Work out the finished part from the listing and answer in its coordinate system (mm). A direction names the side the tool comes from. Round coordinates to 2 decimals unless told otherwise and drop trailing zeros. Order: outer loops, then holes, each group sorted by start corner. A loop starts at its lowest first (then second) coordinate and runs counter-clockwise, first axis right, second up. Notation, with made-up numbers: (35, 46) -> (85, 46) arc R28 cw to (85, 73) -> close; hole circle Ø9 at (4.5, 68). An arc over 180 degrees is marked (long way). Use a Markdown table: item, result. Add a question column.
Item 1: Find the intervals of material crossed by L1, parallel to Z at x = -39, y = -22; L2, parallel to Z at x = -20, y = -17.78; L3, parallel to Z at x = -8.5, y = -53, in increasing order. Write a range as [from, to].
Item 2: A cutting plane is placed at B-B, the plane z = -53.34. Give the number of separate pieces and of enclosed holes in the cut face, plus the area to 3 significant figures.
Item 3: For a pull along X with two mould halves and no side action, classify faces 1 (the flat face through (-38, -28.702, 75)), 2 (the flat face through (-4, -60.757, 1)), 3 (the flat face through (-15.748, -48, -51)), 4 (the cylindrical face through (-41.253, -14.406, 75.323)) as +X half, -X half, draft (parallel to the pull), parting line (faces both ways), or undercut.
Item 4: A cutting plane is placed at A-A, the plane x = -13. Determine the outline of the cut face in (y, z), plus the area to 3 significant figures.
Item 5: A tool of negligible diameter and unlimited length cuts with its end or side. For faces 5 (the cylindrical face through (-8.09, -16.23, -57.08)), 6 (the cylindrical face through (-41.25, -14.41, -69.1)), 7 (the flat face through (-1.524, -30, 78)), from which of +Z, -Z, +X, -X, +Y, -Y can it reach the whole face along a straight path? Write none if from no direction.
Item 6: A cutting plane is placed at C-C, the plane y = -32. Determine the outline of the cut face in (x, z) (3 decimals).
Item 7: Flat-ended cylindrical pins translate along their axes: P1, Ø17, axis at y = -27, z = 72.5, coming from the +X side; P2, Ø9, axis at x = -39.497, z = -74.676, coming from the -Y side; P3, Ø6.5, axis at y = -17.78, z = 48.26, coming from the +X side; P4, Ø1, axis at x = -45, z = 49, coming from the -Y side. Find the tip coordinate at first contact, or state that the pin passes through.
Item 8: A cutting plane is placed at D-D, the plane z = -21.5. Determine the outline of the cut face in (x, y).
from build123d import *

# Parameters (mm, degrees)
EXTRUDE1_DEPTH                              = 95.25
TAPPED_HOLE_FOR_3_8_16_HELICOIL1_AT_2_COUNT = 2
TAPPED_HOLE_FOR_3_8_16_HELICOIL1_AT_2_PITCH = 38.1
TAPPED_HOLE_FOR_3_8_16_HELICOIL1_AT_3_COUNT = 2
TAPPED_HOLE_FOR_3_8_16_HELICOIL1_AT_3_PITCH = 106.3244
TAPPED_HOLE_FOR_3_8_16_HELICOIL1_AT_4_COUNT = 2
TAPPED_HOLE_FOR_3_8_16_HELICOIL1_AT_4_PITCH = 144.4244
TAPPED_HOLE_FOR_1_4_20_HELICOIL1_AT_2_COUNT = 2
TAPPED_HOLE_FOR_1_4_20_HELICOIL1_AT_2_PITCH = 33.02
TAPPED_HOLE_FOR_1_4_20_HELICOIL1_AT_3_COUNT = 2
TAPPED_HOLE_FOR_1_4_20_HELICOIL1_AT_3_PITCH = 106.831083492
TAPPED_HOLE_FOR_1_4_20_HELICOIL1_AT_4_COUNT = 2
TAPPED_HOLE_FOR_1_4_20_HELICOIL1_AT_4_PITCH = 101.6
F_1_4_0_25_DIAMETER_HOLE1_D                 = 6.35
F_1_4_0_25_DIAMETER_HOLE1_CSINK_D           = 7.62
F_1_4_0_25_DIAMETER_HOLE1_CSINK_ANGLE       = 90
SKETCH20_W                                  = 76.2
SKETCH20_H                                  = 60.757213881
SKETCH20_W_2                                = 29.21
SKETCH20_W_3                                = 34.29
EXTRUDE2_DEPTH                              = 1.524


with BuildPart() as part:
    # Sketch13 → Extrude1 (new body, symmetric)
    with BuildSketch(Plane.XY):
        Polygon((0, -60.757213881), (-6.35, -60.757213881), (-76.2, -35.333893017), (-76.2, 0), (0, 0), align=None)
    extrude(amount=EXTRUDE1_DEPTH, both=True)

    # Sketch14 → Tapped Hole for 3/8-16 Helicoil1 (revolve, cut)
    with BuildSketch(Plane(origin=(-39.497, 0, 69.7484), x_dir=(0, 0, 1), z_dir=(1, 0, 0))):
        Polygon((0, 0), (0, 60.757213881), (5.0419, 60.757213881), (5.0419, 28.702), (5.84454, 28.702), (5.84454, 0.50546), (6.35, 0), align=None)
    tapped_hole_for_3_8_16_helicoil1 = revolve(axis=Axis((-39.497, 6.35, 69.7484), (0, -1, 0)), mode=Mode.SUBTRACT)

    # Tapped Hole for 3/8-16 Helicoil1 at 2: Tapped Hole for 3/8-16 Helicoil1 ×2
    with Locations(*[(0, 0, -i * TAPPED_HOLE_FOR_3_8_16_HELICOIL1_AT_2_PITCH) for i in range(1, TAPPED_HOLE_FOR_3_8_16_HELICOIL1_AT_2_COUNT)]):
        add(tapped_hole_for_3_8_16_helicoil1, mode=Mode.SUBTRACT)

    # Tapped Hole for 3/8-16 Helicoil1 at 3: Tapped Hole for 3/8-16 Helicoil1 ×2
    with Locations(*[(0, 0, -i * TAPPED_HOLE_FOR_3_8_16_HELICOIL1_AT_3_PITCH) for i in range(1, TAPPED_HOLE_FOR_3_8_16_HELICOIL1_AT_3_COUNT)]):
        add(tapped_hole_for_3_8_16_helicoil1, mode=Mode.SUBTRACT)

    # Tapped Hole for 3/8-16 Helicoil1 at 4: Tapped Hole for 3/8-16 Helicoil1 ×2
    with Locations(*[(0, 0, -i * TAPPED_HOLE_FOR_3_8_16_HELICOIL1_AT_4_PITCH) for i in range(1, TAPPED_HOLE_FOR_3_8_16_HELICOIL1_AT_4_COUNT)]):
        add(tapped_hole_for_3_8_16_helicoil1, mode=Mode.SUBTRACT)

    # Sketch16 → Tapped Hole for 1/4-20 Helicoil1 (revolve, cut)
    with BuildSketch(Plane(origin=(0, -17.78, 48.26), x_dir=(0, 0, -1), z_dir=(0, 1, 0))):
        Polygon((0, 0), (0, 25.905827343), (3.3782, 23.876), (3.3782, 15.748), (4.04749, 15.748), (4.04749, 0.635), (4.68249, 0), align=None)
    tapped_hole_for_1_4_20_helicoil1 = revolve(axis=Axis((6.35, -17.78, 48.26), (-1, 0, 0)), mode=Mode.SUBTRACT)

    # Tapped Hole for 1/4-20 Helicoil1 at 2: Tapped Hole for 1/4-20 Helicoil1 ×2
    with Locations(*[(0, -i * TAPPED_HOLE_FOR_1_4_20_HELICOIL1_AT_2_PITCH, 0) for i in range(1, TAPPED_HOLE_FOR_1_4_20_HELICOIL1_AT_2_COUNT)]):
        add(tapped_hole_for_1_4_20_helicoil1, mode=Mode.SUBTRACT)

    # Tapped Hole for 1/4-20 Helicoil1 at 3: Tapped Hole for 1/4-20 Helicoil1 ×2
    with Locations(*[Vector(0, -0.309086072, -0.951034069) * (i * TAPPED_HOLE_FOR_1_4_20_HELICOIL1_AT_3_PITCH) for i in range(1, TAPPED_HOLE_FOR_1_4_20_HELICOIL1_AT_3_COUNT)]):
        add(tapped_hole_for_1_4_20_helicoil1, mode=Mode.SUBTRACT)

    # Tapped Hole for 1/4-20 Helicoil1 at 4: Tapped Hole for 1/4-20 Helicoil1 ×2
    with Locations(*[(0, 0, -i * TAPPED_HOLE_FOR_1_4_20_HELICOIL1_AT_4_PITCH) for i in range(1, TAPPED_HOLE_FOR_1_4_20_HELICOIL1_AT_4_COUNT)]):
        add(tapped_hole_for_1_4_20_helicoil1, mode=Mode.SUBTRACT)

    # 1/4 (0.25) Diameter Hole1 (through all)
    with Locations(Plane(origin=(0, 0, 0), x_dir=(-1, 0, 0), z_dir=(0, 1, 0))):
        with Locations((23.876, -53.34), (23.876, 48.26)):
            CounterSinkHole(F_1_4_0_25_DIAMETER_HOLE1_D / 2, F_1_4_0_25_DIAMETER_HOLE1_CSINK_D / 2, counter_sink_angle=F_1_4_0_25_DIAMETER_HOLE1_CSINK_ANGLE)

    # Sketch20 → Extrude2 (cut)
    with BuildSketch(Plane(origin=(0, 0, 0), x_dir=(0, 0, -1), z_dir=(1, 0, 0))):
        with Locations((2.54, -30.378606941)):
            Rectangle(SKETCH20_W, SKETCH20_H)
        with Locations((80.645, -30.378606941)):
            Rectangle(SKETCH20_W_2, SKETCH20_H)
        with Locations((-78.105, -30.378606941)):
            Rectangle(SKETCH20_W_3, SKETCH20_H)
    extrude(amount=-EXTRUDE2_DEPTH, mode=Mode.SUBTRACT)


solid = part.part
Reported:
| question | item | result |
|---|---|---|
| 1 | L1 | [-95.25, -80.5], [-68.85, -42.4], [-30.75, 25.83], [37.47, 63.93], [75.57, 95.25] |
| 1 | L2 | [-95.25, -56.72], [-49.96, 44.88], [51.64, 95.25] |
| 1 | L3 | [-95.25, -56.74], [-49.94, 44.86], [51.66, 95.25] |
| 2 | separate pieces | 4 |
| 2 | enclosed holes | 0 |
| 2 | area | 3,070 mm² |
| 3 | face 1 | undercut |
| 3 | face 2 | draft |
| 3 | face 3 | +X half |
| 3 | face 4 | undercut |
| 4 | outline | (-58.34, -95.25) -> (0, -95.25) -> (0, 95.25) -> (-58.34, 95.25) -> close; hole circle Ø8.09 at (-50.8, -53.34); hole circle Ø8.09 at (-50.8, 48.26); hole circle Ø8.09 at (-17.78, -53.34); hole circle Ø8.09 at (-17.78, 48.26) |
| 4 | area | 10,900 mm² |
| 5 | face 5 | +X |
| 5 | face 6 | +Y |
| 5 | face 7 | +Z, +X, +Y, -Y |
| 6 | outline | (-76.2, -95.25) -> (-1.524, -95.25) -> (-1.524, -66.04) -> (0, -66.04) -> (0, -40.64) -> (-1.524, -40.64) -> (-1.524, 35.56) -> (0, 35.56) -> (0, 60.96) -> (-1.524, 60.96) -> (-1.524, 95.25) -> (-76.2, 95.25) -> close; hole circle Ø10.084 at (-39.497, -74.676); hole circle Ø10.084 at (-39.497, -36.576); hole circle Ø10.084 at (-39.497, 31.648); hole circle Ø10.084 at (-39.497, 69.748); hole circle Ø6.35 at (-23.876, -53.34); hole circle Ø6.35 at (-23.876, 48.26) |
| 7 | P1 | x = -1.52 |
| 7 | P2 | through |
| 7 | P3 | x = -23.95 |
| 7 | P4 | y = -46.87 |
| 8 | outline | (-76.2, -35.33) -> (-6.35, -60.76) -> (-1.52, -60.76) -> (-1.52, 0) -> (-76.2, 0) -> close |
